Verification items for the finished model (mm, model axes). A direction names the side the tool comes from. Give positions to 0.01 mm unless a question says otherwise; leave off trailing zeros. Loops run counter-clockwise (first coordinate to the right, second up) from the corner with the lowest first, then second, coordinate; pieces in that order, holes last. Notation, with made-up numbers: (35, 84.25) - (79, 84.25) arc R10 cw to (79, 100.25) - close; hole circle Ø9 at (-36.5, 7.5). An arc over 180 degrees is marked (long way). One line per item, written item: value. Start each with the question number.
1. Sectioned sample at B-B (z = 20.5). Record the cut outline in (x, y), plus the area to 3 significant figures.
2. Scan lines: L1, parallel to Y at x = 0, z = 13.5; L2, parallel to Y at x = -2.25, z = 26.5; L3, parallel to X at y = 2, z = 9. Record each from-to range of solid material in increasing order. Write a range as [from, to].
3. Mould release check, pull along X, two halves, no side actions. Record for faces 3 (the cylindrical face through (-1.886, -8.493, 19.72)), 4 (the flat face through (9.2, 5.9, 19)), 5 (the cylindrical face through (-1.4, 10.66, 9.37)): pulls with the +X half, pulls with the -X half, needs draft (parallel to the pull), parting line crosses it, or undercut.
4. Access from +Z, -Z, +X, -X, +Y, -Y to the whole of each face (thin tool, end or side, straight path). Record for faces 1 (the conical face through (10.543, 3.32, 29.647)), 2 (the flat face through (-1, -9, 40)).
5. Gauge pin test, flat ends, axial feed: pin 1 (8 mm diameter, centred on x = 3.5, z = 23, fed in from -Y); pin 2 (10 mm diameter, centred on x = -1.5, z = 35, fed in from +Y); pin 3 (10 mm diameter, centred on x = 6.5, z = 8, fed in from +Y). Record the tip position at first contact, or that the pin passes through.
6. Sectioned sample at A-A (z = 11). Record the cut outline in (x, y).
from build123d import *

# Parameters (mm, degrees)
CYLINDER005_R     = 8.7
CYLINDER005_DEPTH = 40
CYLINDER007_R     = 10.75
CYLINDER007_DEPTH = 40


with BuildPart() as outletextension:
    # Cylinder005 → Cylinder005 (new body)
    with BuildSketch(Plane.XY):
        Circle(CYLINDER005_R)
    extrude(amount=CYLINDER005_DEPTH)


with BuildPart() as housingoutlet:
    # Cylinder007 → Cylinder007 (new body)
    with BuildSketch(Plane.XY):
        Circle(CYLINDER007_R)
    extrude(amount=CYLINDER007_DEPTH)


with BuildPart() as bloweroutletadapter_v3:
    # Cone001 → Cone001 (revolve)
    with BuildSketch(Plane(origin=(0, 0, 19), x_dir=(1, 0, 0), z_dir=(0, -1, 0))):
        Polygon((0, 0), (11.19, 0), (10.92, 21), (0, 21), align=None)
    revolve(axis=Axis((0, 0, 19), (0, 0, 1)))

    # Fusion: union HousingOutlet
    add(housingoutlet.part)

    # Cut: cut OutletExtension
    add(outletextension.part, mode=Mode.SUBTRACT)


solid = bloweroutletadapter_v3.part
Results are:
1. outline: circle Ø22.34 at (0, 0); hole circle Ø17.4 at (0, 0)
1. area: 154 mm^2
2. L1: y = [-10.75, -8.7], [8.7, 10.75]
2. L2: y = [-10.86, -8.4], [8.4, 10.86]
2. L3: x = [-10.56, -8.47], [8.47, 10.56]
3. face 3: undercut
3. face 4: needs draft
3. face 5: parting line crosses it
4. face 1: +Z
4. face 2: +Z, +X, -X, +Y, -Y
5. pin 1: stops at y = -11.17
5. pin 2: stops at y = 11.05
5. pin 3: stops at y = 10.64
6. outline: circle Ø21.5 at (0, 0); hole circle Ø17.4 at (0, 0)
